The listing builds one solid part. Answer for the finished solid, in the listing's coordinates (mm). Coordinates: 2 decimals unless noted, no trailing zeros. Loops run counter-clockwise (first coordinate to the right, second up) from the corner with the lowest first, then second, coordinate; pieces in that order, holes last. Notation, with made-up numbers: M -34.5,33.25 L 10.5,33.25 A22 cw 10.5,54.25 Z; hole C 29.5,76.25 d3. An arc over 180 degrees is marked long. Answer in a Markdown table with one row per item. Add a question column.
from build123d import *

# Parameters (mm, degrees)
SKETCH036_W = 12
SKETCH036_H = 0.5


with BuildPart() as washer:
    # Sketch036 → Revolution001 (revolve)
    with BuildSketch(Plane.XY):
        with Locations((-18.5, 5.75)):
            Rectangle(SKETCH036_W, SKETCH036_H)
    revolve(axis=Axis((0, 0, 0), (1, 0, 0)))


with BuildPart() as washer_1:
    # Body008 placement: moved
    add(washer.part.moved(Location((0, -51, -44))))


with BuildPart() as part_mirroring006:
    # Part__Mirroring006: instance of washer
    add(washer_1.part.mirror(Plane(origin=(0, 0, 0), x_dir=(0, -1, 0), z_dir=(1, 0, 0))))


with BuildPart() as part_mirroring007:
    # Part__Mirroring007: instance of Part__Mirroring006
    add(part_mirroring006.part.mirror(Plane(origin=(0, 0, 0), x_dir=(1, 0, 0), z_dir=(0, 1, 0))))


with BuildPart() as part_mirroring008:
    # Part__Mirroring008: instance of Part__Mirroring007
    add(part_mirroring007.part.mirror(Plane(origin=(0, 0, 0), x_dir=(0, -1, 0), z_dir=(1, 0, 0))))


solid = part_mirroring008.part
(1) A cutting plane is placed at B-B (z = -44). Give the vertices of the cut face in (x, y).
(2) A cutting plane is placed at C-C (x = -14.75). Give the vertices of the cut face in (y, z), plus the area to 3 significant figures.
(3) A cutting plane is placed at A-A (y = 51). Give the vertices of the cut face in (x, z), plus the area to 3 significant figures.
(4) The mould has two halves that part along Y. Classify faces 1 (the face through (-18.416, 56.495, -43.758)), 2 (the face through (-24.5, 56, -47)), 3 (the face through (-18.416, 52.301, -49.857)): released by +Y, released by -Y, zero draft, split by the parting line, or undercut.
(5) Straight lines are drawn through the part: line 1 (Z direction, x = -18.5, y = 51); line 2 (Z direction, x = -21, y = 54.25); line 3 (Y direction, x = -21.25, z = -48.5). For each, find the intervals that lie inside material, in ascending order.
(6) Each of these flat-tipped pins is pushed along its axis until it touches: pin 1 (4 mm diameter, centred on x = -15.5, y = 53.5, fed in from +Z); pin 2 (1 mm diameter, centred on x = -20, y = 54.5, fed in from +Z); pin 3 (1.5 mm diameter, centred on x = -19.5, z = -46, fed in from +Y); pin 4 (4 mm diameter, centred on y = 48, z = -44, fed in from +X) (1 decimal). Where does it stop, or does it pass through?
Solved:
| question | item | result |
|---|---|---|
| 1 | outline | M -24.5,45 L -12.5,45 L -12.5,45.5 L -24.5,45.5 Z; M -24.5,56.5 L -12.5,56.5 L -12.5,57 L -24.5,57 Z |
| 2 | outline | C 51,-44 d12; hole C 51,-44 d11 |
| 2 | area | 18.1 mm² |
| 3 | outline | M -24.5,-50 L -12.5,-50 L -12.5,-49.5 L -24.5,-49.5 Z; M -24.5,-38.5 L -12.5,-38.5 L -12.5,-38 L -24.5,-38 Z |
| 3 | area | 12.0 mm² |
| 4 | face 1 | undercut |
| 4 | face 2 | zero draft |
| 4 | face 3 | split by the parting line |
| 5 | line 1 | z = -50 to -49.5, -38.5 to -38 |
| 5 | line 2 | z = -49.04 to -48.44, -39.56 to -38.96 |
| 5 | line 3 | y = 47.03 to 47.84, 54.16 to 54.97 |
| 6 | pin 1 | stops at z = -38.02 |
| 6 | pin 2 | stops at z = -38.8 |
| 6 | pin 3 | stops at y = 56.87 |
| 6 | pin 4 | passes through |
